Check sheet for the modelled part. Datum: model origin and axes. Units: mm. Round coordinates to 2 decimals unless told otherwise and drop trailing zeros. Loops run counter-clockwise (first coordinate to the right, second up) from the corner with the lowest first, then second, coordinate; pieces in that order, holes last. Notation, with made-up numbers: (71.5, 41) -> (120.5, 41) arc R12 ccw to (120.5, 59) -> close; hole circle Ø2 at (42.5, -11.5). An arc over 180 degrees is marked (long way). One line per item, written item: value. Start each with the question number.
1. Cross-section at B-B on z = -3.25. Record the cut outline in (x, y).
2. Cross-section at A-A on y = 15. Record the cut outline in (x, z) (3 decimals).
3. Cross-section at D-D on z = -15. Record the cut outline in (x, y) (3 decimals).
4. Material ranges on L1, parallel to Y at x = 3.5, z = -15 (3 decimals); L2, parallel to Z at x = 5.5, y = 2.84; L3, parallel to Y at x = 5, z = -3, recorded low to high.
5. Go/stop test with flat-tipped pins: pin 1 (4 mm diameter, centred on y = 2.84, z = -27, fed in from +X); pin 2 (1.9 mm diameter, centred on y = 27.16, z = -3, fed in from +X). Record where each tip stops, or that it passes through.
6. Cross-section at C-C on x = 5.5. Count the separate pieces of the cut face and the enclosed holes in it, then the cut area to 3 significant figures.
7. Release check for a two-part mould opening along Z. For faces 1 (the face through (4, 15, 0)), 2 (the face through (4, 30, -15)), 3 (the face through (3.757, 3.448, -28.466)) record: +Z half, -Z half, draft (parallel to the pull), parting line (faces both ways), or undercut.
Autodesk Inventor part; units mm, degrees
ref_plane "YZ Plane" through (0, 0, 0) normal (1, 0, 0) x (0, 1, 0)
ref_plane "XZ Plane" through (0, 0, 0) normal (0, 1, 0) x (-1, 0, 0)
ref_plane "XY Plane" through (0, 0, 0) normal (0, 0, 1) x (1, 0, 0)
sketch "Sketch1" plane through (0, 0, 0) normal (1, 0, 0) x (0, 1, 0)
  line L0 (0, 0) -> (30, 0)
  line L1 (30, 0) -> (30, -30)
  line L2 (30, -30) -> (0, -30)
  line L3 (0, -30) -> (0, 0)
  dimension "d0" = 30
  dimension "d1" = 30
extrude "Extrusion1" add sketch "Sketch1" along normal blind 7.62
sketch "Sketch2" plane through (7.62, 0, 0) normal (1, 0, 0) x (0, 0, -1)
  line L0 (0, 30) -> (0, 0)
  line L1 (0, 0) -> (30, 0)
  line L2 (30, 0) -> (30, 30)
  line L3 (30, 30) -> (0, 30)
  line L4 (15, 30) -> (15, 0) construction
  line L5 (0, 15) -> (30, 15) construction
  circle A0 centre (15, 15) radius 14.225
  dimension "d4" = 28.45
extrude "Extrusion2" cut sketch "Sketch2" against normal blind 7.62 contours A0
sketch "Sketch3" plane through (7.62, 0, 0) normal (1, 0, 0) x (0, 0, -1)
  line L0 (0, 30) -> (30, 30) construction
  line L1 (15, 30) -> (15, 0) construction
  line L2 (30, 0) -> (0, 0) construction
  line L3 (0, 0) -> (0, 30) construction
  line L4 (0, 15) -> (29.023, 15) construction
  point P0 (3, 2.84)
  point P1 (3, 27.16)
  point P2 (27, 2.84)
  point P3 (27, 27.16)
  dimension "d15" = 2.84
hole "Hole1" at (7.62, 2.84, -3) at (7.62, 27.16, -3) at (7.62, 27.16, -27) at (7.62, 2.84, -27) direction (-1, 0, 0) diameter 3.175 end through all
properties part number "Pi Fan" material "PPS Plastic"
Taken from the geometry:
1. outline: (0, 0) -> (7.62, 0) -> (7.62, 1.27) -> (0, 1.27) -> close; (0, 4.41) -> (7.62, 4.41) -> (7.62, 6.98) -> (0, 6.98) -> close; (0, 23.02) -> (7.62, 23.02) -> (7.62, 25.59) -> (0, 25.59) -> close; (0, 28.73) -> (7.62, 28.73) -> (7.62, 30) -> (0, 30) -> close
2. outline: (0, -30) -> (7.62, -30) -> (7.62, -29.225) -> (0, -29.225) -> close; (0, -0.775) -> (7.62, -0.775) -> (7.62, 0) -> (0, 0) -> close
3. outline: (0, 0) -> (7.62, 0) -> (7.62, 0.775) -> (0, 0.775) -> close; (0, 29.225) -> (7.62, 29.225) -> (7.62, 30) -> (0, 30) -> close
4. L1: y = 0 to 0.775, 29.225 to 30
4. L2: z = -30 to -28.59, -25.41 to -22.38, -7.62 to -4.59, -1.41 to 0
4. L3: y = 0 to 1.25, 4.43 to 7.36, 22.64 to 25.57, 28.75 to 30
5. pin 1: stops at x = 7.62
5. pin 2: passes through
6. separate pieces: 1
6. enclosed holes: 5
6. area: 233 mm2
7. face 1: +Z half
7. face 2: draft
7. face 3: undercut
